Input: dimensioned drawing with shaded views. Units: mm. Origin: part minimum x, y, z. A direction names the side the tool comes from. Give positions to 0.01 mm unless a question says otherwise; leave off trailing zeros. Write each loop counter-clockwise with the first axis right and the second up, starting at its lowest first coordinate (ties: lowest second). Pieces come first, ordered by that corner, then holes.
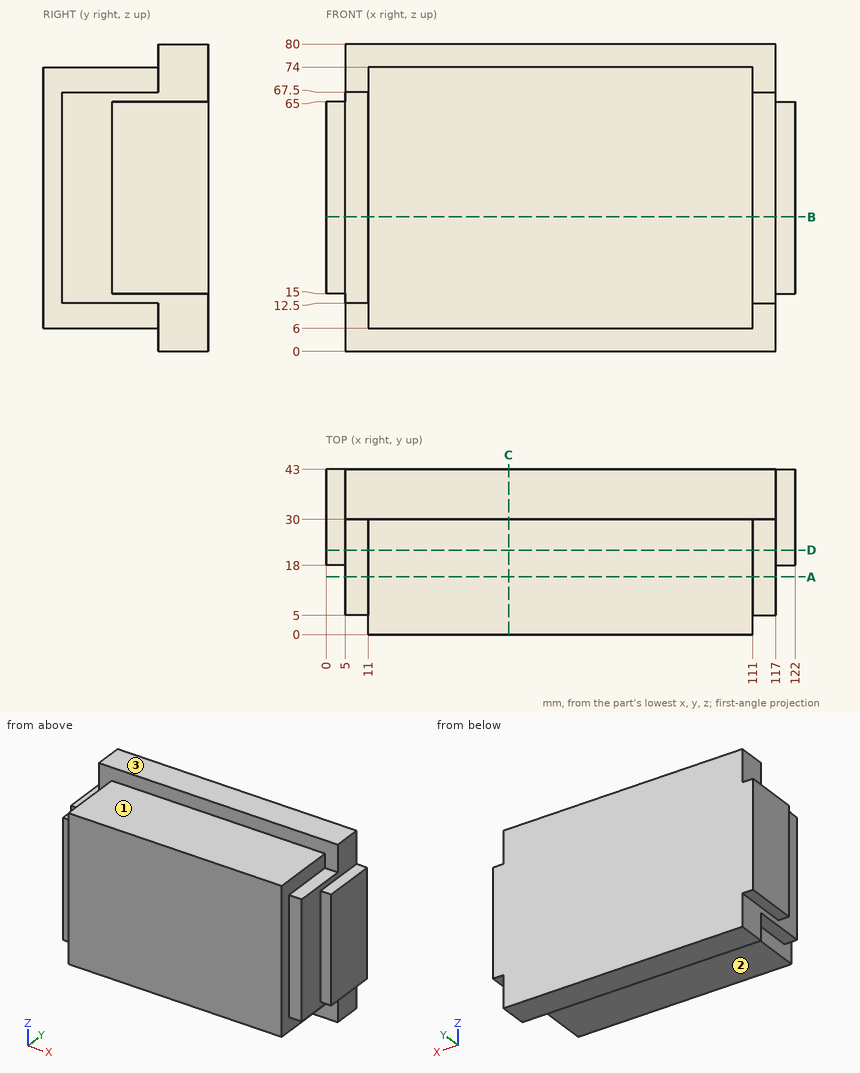
Item 1: Section A-A, the plane y = 15. Return the cut outline in (x, z), plus the area to 3 significant figures.
Found:
outline: (5, 12.5) - (11, 12.5) - (11, 6) - (111, 6) - (111, 12.5) - (117, 12.5) - (117, 67.5) - (111, 67.5) - (111, 74) - (11, 74) - (11, 67.5) - (5, 67.5) - close
area: 7,460 mm2
Item 2: Section B-B, the plane z = 35. Return the cut outline in (x, y).
Found:
outline: (0, 18) - (5, 18) - (5, 5) - (11, 5) - (11, 0) - (111, 0) - (111, 5) - (117, 5) - (117, 18) - (122, 18) - (122, 43) - (0, 43) - close
Item 3: Reachability of the marked faces 1, 2 and 3 from +Z, -Z, +X, -X, +Y, -Y: full face, straight path, thin tool, end or side. Return the list, or none.
Found:
face 1: +Z, +X, -X, -Y
face 2: -Z, +X, -X, -Y
face 3: +Z, +X, -X, +Y, -Y
Item 4: Section C-C, the plane x = 47.5. Return the cut outline in (y, z), plus the area to 3 significant figures.
Found:
outline: (0, 6) - (30, 6) - (30, 0) - (43, 0) - (43, 80) - (30, 80) - (30, 74) - (0, 74) - close
area: 3,080 mm2
Item 5: Section D-D, the plane y = 22. Return the cut outline in (x, z).
Found:
outline: (0, 15) - (5, 15) - (5, 12.5) - (11, 12.5) - (11, 6) - (111, 6) - (111, 12.5) - (117, 12.5) - (117, 15) - (122, 15) - (122, 65) - (117, 65) - (117, 67.5) - (111, 67.5) - (111, 74) - (11, 74) - (11, 67.5) - (5, 67.5) - (5, 65) - (0, 65) - close
Item 6: Line query: L1, parallel to Y at x = 112, z = 39; L2, parallel to Z at x = 21, y = 15.5; L3, parallel to X at y = 12.5, z = 54. Output: solid intervals per line, ascending.
Found:
L1: y = 5 to 43
L2: z = 6 to 74
L3: x = 5 to 117
Item 7: Pin query (flat end, axial travel): pin 1 Ø6.5 at (x, y) = (9.5, 17) entering from -Z; pin 2 Ø6.5 at (x, y) = (114.5, 19.5) entering from -Z; pin 3 Ø5.5 at (x, z) = (120.5, 34) entering from -Y. Return the tip coordinate at first contact, or that it passes through.
Found:
pin 1: stops at z = 6
pin 2: stops at z = 12.5
pin 3: stops at y = 18
